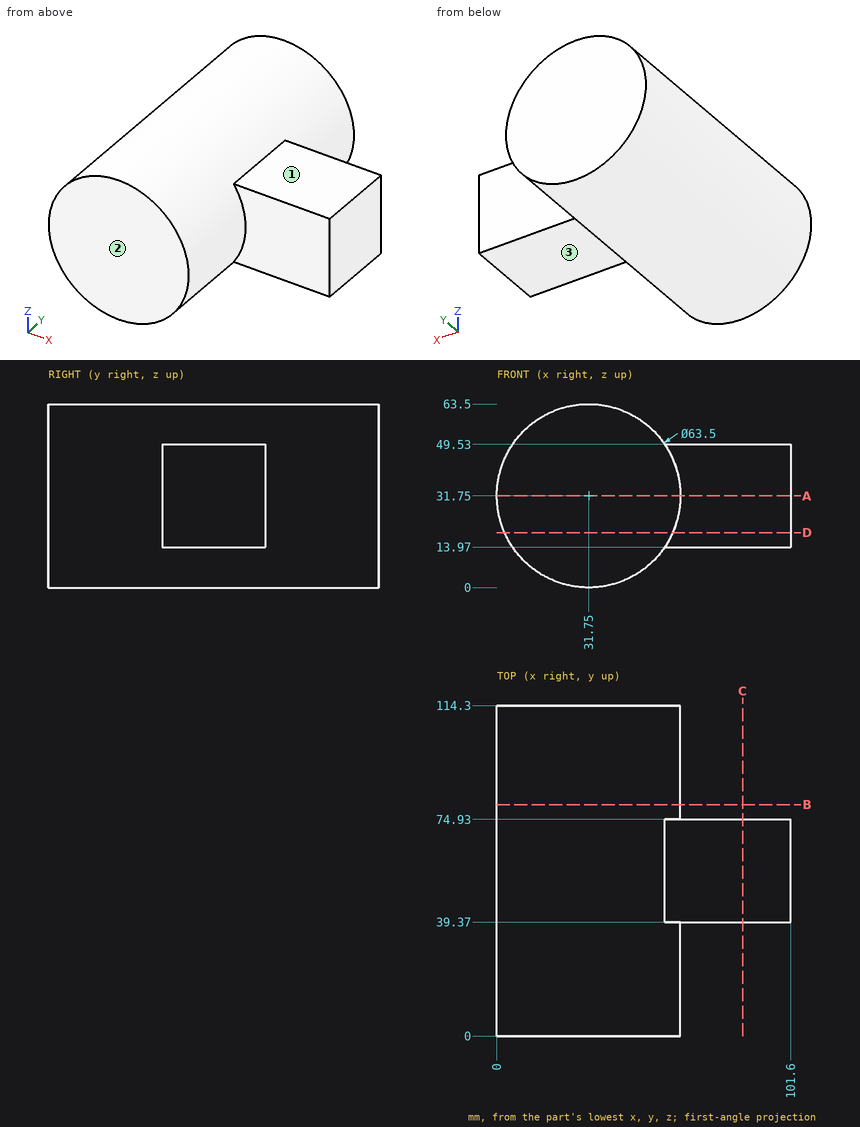
Study the drawing (mm; zero at the part's minimum x, y, z) and answer. A direction names the side the tool comes from. Coordinates: 2 decimals unless noted, no trailing zeros. Write each loop counter-clockwise with the first axis right and the second up, starting at its lowest first coordinate (ties: lowest second). Pieces come first, ordered by that corner, then holes. Notation, with made-up numbers: M 6.5,13.5 L 57.5,13.5 A29 ccw 57.5,44.5 Z; hole C 36,-7.75 d4. An arc over 180 degrees is marked long. Use a Markdown table: item, result. Add a question column.
1. Section A-A (z = 31.75) is taken. Give the vertices of the cut face in (x, y).
2. Section C-C (x = 85) is taken. Give the vertices of the cut face in (y, z), plus the area to 3 significant figures.
3. Straight lines are drawn through the part: line 1 along X through (y, z) = (86, 32); line 2 along X through (y, z) = (56.5, 31.5); line 3 along Z through (x, y) = (90.5, 62.5). For each, find the intervals that lie inside material, in ascending order. Write a range as [from, to].
4. Section B-B (y = 80) is taken. Give the vertices of the cut face in (x, z).
5. Given P1, Ø10.5, axis at x = 78, y = 58.5, coming from the -Z side; P2, Ø8, axis at y = 93.5, z = 56, coming from the +X side; P3, Ø8, axis at x = 65, z = 46.5, coming from the -Y side, each flat-ended and moving along its own axis, determine where each tip first touches the part or whether it passes through.
6. Section D-D (z = 19) is taken. Give the vertices of the cut face in (x, y), plus the area to 3 significant figures.
7. Which of the six approach directions +Z, -Z, +X, -X, +Y, -Y give full straight-line access (tool end or side, diameter ignored) to the marked faces 1, 2 and 3?
Data:
| question | item | result |
|---|---|---|
| 1 | outline | M 0,0 L 63.5,0 L 63.5,39.37 L 101.6,39.37 L 101.6,74.93 L 63.5,74.93 L 63.5,114.3 L 0,114.3 Z |
| 2 | outline | M 39.37,13.97 L 74.93,13.97 L 74.93,49.53 L 39.37,49.53 Z |
| 2 | area | 1,260 mm2 |
| 3 | line 1 | x = [0, 63.5] |
| 3 | line 2 | x = [0, 101.6] |
| 3 | line 3 | z = [13.97, 49.53] |
| 4 | outline | C 31.75,31.75 d63.5 |
| 5 | P1 | stops at z = 13.97 |
| 5 | P2 | stops at x = 56.2 |
| 5 | P3 | stops at y = 39.37 |
| 6 | outline | M 2.67,0 L 60.83,0 L 60.83,39.37 L 101.6,39.37 L 101.6,74.93 L 60.83,74.93 L 60.83,114.3 L 2.67,114.3 Z |
| 6 | area | 8,100 mm2 |
| 7 | face 1 | +Z, +X, +Y, -Y |
| 7 | face 2 | +Z, -Z, +X, -X, -Y |
| 7 | face 3 | -Z, +X, +Y, -Y |
